```python
from build123d import *

# Parameters (mm, degrees)
SKETCH_1_R          = 3.515
EXTRUDE_1_DEPTH     = 4
FILLET_1_R          = 10
SKETCH_3_R          = 4.15
CUT_EXTRUDE_2_DEPTH = 0.1
CUT_EXTRUDE_START   = -0.1
SKETCH_4_R          = 4.15
CUT_EXTRUDE_3_DEPTH = 0.1


with BuildPart() as part:
    # 草图1 → 凸台-拉伸1 (new body)
    with BuildSketch(Plane(origin=(0, 0, 0), x_dir=(1, 0, 0), z_dir=(0, 1, 0))):
        with BuildLine():
            Line((4.898979486, 2.5), (115.101020514, 2.5))
            ThreePointArc((115.101020514, 2.5), (125.5, 0), (115.101020514, -2.5))
            Line((115.101020514, -2.5), (4.898979486, -2.5))
            ThreePointArc((4.898979486, -2.5), (-5.5, 0), (4.898979486, 2.5))
        make_face()
        with Locations(Location((0, 0, 0), (0, 0, 270))):
            Circle(SKETCH_1_R, mode=Mode.SUBTRACT)
        with Locations(Location((120, 0, 0), (0, 0, 270))):
            Circle(SKETCH_1_R, mode=Mode.SUBTRACT)
    extrude(amount=EXTRUDE_1_DEPTH)

    # 圆角1
    fillet_1_edges = [part.edges().sort_by_distance(p)[0] for p in [
        (4.898979486, 2, -2.5),
        (115.101020514, 2, -2.5),
        (115.101020514, 2, 2.5),
        (4.898979486, 2, 2.5),
    ]]
    fillet(fillet_1_edges, radius=FILLET_1_R)

    # 草图3 → 切除-拉伸2 (cut)
    with BuildSketch(Plane(origin=(0, 4, 0), x_dir=(1, 0, 0), z_dir=(0, 1, 0))):
        with Locations(Location((0, 0, 0), (0, 0, 270))):
            Circle(SKETCH_3_R)
        with Locations(Location((120, 0, 0), (0, 0, 270))):
            Circle(SKETCH_3_R)
    extrude(amount=-CUT_EXTRUDE_2_DEPTH, mode=Mode.SUBTRACT)

    # 草图4 → 切除-拉伸3 (cut)
    with BuildSketch(Plane.XZ.offset(CUT_EXTRUDE_START)):
        with Locations(Location((0, 0, 0), (0, 0, 90))):
            Circle(SKETCH_4_R)
        with Locations(Location((120, 0, 0), (0, 0, 90))):
            Circle(SKETCH_4_R)
    extrude(amount=CUT_EXTRUDE_3_DEPTH, mode=Mode.SUBTRACT)


solid = part.part
```
Source: CAD feature listing. Evaluate the final solid. Frame: model axes, mm. A direction names the side the tool comes from. Round coordinates to 2 decimals unless told otherwise and drop trailing zeros. Loops run counter-clockwise (first coordinate to the right, second up) from the corner with the lowest first, then second, coordinate; pieces in that order, holes last.
1. Section query A-A on x = 0. Output: boundary loops of the cut face in (y, z) (3 decimals), and give its area (3 significant figures).
2. Contact query for flat-ended pins moving along their axis: pin 1 (2 mm diameter, centred on y = 0.5, z = 3, fed in from -X); pin 2 (4 mm diameter, centred on x = 0, z = 0, fed in from -Y); pin 3 (2 mm diameter, centred on y = 2.5, z = 4, fed in from -X); pin 4 (1.2 mm diameter, centred on x = 49.5, y = 3, fed in from -Z). Output: stop coordinate, or through.
3. Ray query, L1, parallel to X at y = 1.7, z = 0 (3 decimals); L2, parallel to X at y = 1.4, z = 2; L3, parallel to Z at x = 78, y = 3.6. Return the intervals inside material, ascending.
4. Access query for faces 4 (the cylindrical face through (113.9, 2.03, -2.98)), 5 (the flat face through (61, 4, 0)), 6 (the cylindrical face through (113.99, 2.03, 3.01)). Directions: +Z, -Z, +X, -X, +Y, -Y. A direction counts if a zero-diameter tool reaches every point of the face in a straight line with its end or side. Return the directions, or none.
5. Section query C-C on y = 3. Output: boundary loops of the cut face in (x, z) (3 decimals).
6. Section query D-D on x = 81. Output: boundary loops of the cut face in (y, z), and give its area (3 significant figures).
7. Mould query, pull axis Z, two halves, no side actions, for faces 1 (the flat face through (59, 2, -2.5)), 2 (the flat face through (61, 2, 2.5)), 3 (the cylindrical face through (116.57, 1.97, -0.76)). Classes: released by +Z, released by -Z, zero draft, split by the parting line, or undercut.
8. Section query B-B on z = 0. Output: boundary loops of the cut face in (x, y) (3 decimals), and give its area (3 significant figures).
Answers below:
1. outline: (0, -5.5) - (4, -5.5) - (4, -4.15) - (3.9, -4.15) - (3.9, -3.515) - (0.1, -3.515) - (0.1, -4.15) - (0, -4.15) - close; (0, 4.15) - (0.1, 4.15) - (0.1, 3.515) - (3.9, 3.515) - (3.9, 4.15) - (4, 4.15) - (4, 5.5) - (0, 5.5) - close
1. area: 15.6 mm2
2. pin 1: stops at x = -5.12
2. pin 2: passes through
2. pin 3: stops at x = -4.61
2. pin 4: stops at z = -2.5
3. L1: x = -5.5 to -3.515, 3.515 to 116.485, 123.515 to 125.5
3. L2: x = -5.12 to -2.89, 2.89 to 117.11, 122.89 to 125.12
3. L3: z = -2.5 to 2.5
4. face 4: -Z, +Y, -Y
4. face 5: +Z, -Z, +X, -X, +Y
4. face 6: +Z, +Y, -Y
5. outline: (3.252, -4.435) arc R10 cw to (9.165, -2.5) - (110.835, -2.5) arc R10 cw to (116.748, -4.435) arc R5.5 ccw (long way) to (116.748, 4.435) arc R10 cw to (110.835, 2.5) - (9.165, 2.5) arc R10 cw to (3.252, 4.435) arc R5.5 ccw (long way) to start; hole circle Ø7.03 at (0, 0); hole circle Ø7.03 at (120, 0)
6. outline: (0, -2.5) - (4, -2.5) - (4, 2.5) - (0, 2.5) - close
6. area: 20.0 mm2
7. face 1: released by -Z
7. face 2: released by +Z
7. face 3: undercut
8. outline: (-5.5, 0) - (-4.15, 0) - (-4.15, 0.1) - (-3.515, 0.1) - (-3.515, 3.9) - (-4.15, 3.9) - (-4.15, 4) - (-5.5, 4) - close; (3.515, 0.1) - (4.15, 0.1) - (4.15, 0) - (115.85, 0) - (115.85, 0.1) - (116.485, 0.1) - (116.485, 3.9) - (115.85, 3.9) - (115.85, 4) - (4.15, 4) - (4.15, 3.9) - (3.515, 3.9) - close; (123.515, 0.1) - (124.15, 0.1) - (124.15, 0) - (125.5, 0) - (125.5, 4) - (124.15, 4) - (124.15, 3.9) - (123.515, 3.9) - close
8. area: 467 mm2
